from build123d import *

# Parameters (mm, degrees)
SKETCH_1_R          = 2
SKETCH_1_R_2        = 1.5
SKETCH_1_R_3        = 13.75
EXTRUDE_1_DEPTH     = 4
SKETCH1_W           = 111
SKETCH1_H           = 110
SKETCH1_R           = 1.6
SKETCH1_R_2         = 2.1
SKETCH1_R_3         = 25
BOSS_EXTRUDE1_DEPTH = 4
FILLET1_R           = 10
FILLET2_DEPTH       = 4
CUT_EXTRUDE1_DEPTH  = 10


with BuildPart() as part:
    # 草图1 → 凸台-拉伸1 (new body)
    with BuildSketch(Plane(origin=(0, 0, 0), x_dir=(1, 0, 0), z_dir=(0, 1, 0))):
        with BuildLine():
            Line((-43.799718629, 20.922806374), (-13.545390598, 30.755183267))
            ThreePointArc((-13.545390598, 30.755183267), (-12.782331025, 30.938416565), (-12, 31))
            Line((-12, 31), (12, 31))
            ThreePointArc((12, 31), (12.782331025, 30.938416565), (13.545390598, 30.755183267))
            Line((13.545390598, 30.755183267), (43.799718629, 20.922806374))
            ThreePointArc((43.799718629, 20.922806374), (58.729032885, -3.442256511), (37, -22))
            Line((37, -22), (-37, -22))
            ThreePointArc((-37, -22), (-58.729032885, -3.442256511), (-43.799718629, 20.922806374))
        make_face()
        with Locations(Location((-12, 26, 0), (0, 0, 270))):
            Circle(SKETCH_1_R, mode=Mode.SUBTRACT)
        with Locations(Location((12, 26, 0), (0, 0, 270))):
            Circle(SKETCH_1_R, mode=Mode.SUBTRACT)
        with Locations(Location((49.374368671, 12.374368671, 0), (0, 0, 270))):
            Circle(SKETCH_1_R_2, mode=Mode.SUBTRACT)
        with Locations(Location((49.374368671, -12.374368671, 0), (0, 0, 270))):
            Circle(SKETCH_1_R_2, mode=Mode.SUBTRACT)
        with Locations(Location((24.625631329, -12.374368671, 0), (0, 0, 270))):
            Circle(SKETCH_1_R_2, mode=Mode.SUBTRACT)
        with Locations(Location((24.625631329, 12.374368671, 0), (0, 0, 270))):
            Circle(SKETCH_1_R_2, mode=Mode.SUBTRACT)
        with Locations(Location((-49.374368671, -12.374368671, 0), (0, 0, 90))):
            Circle(SKETCH_1_R_2, mode=Mode.SUBTRACT)
        with Locations(Location((-24.625631329, -12.374368671, 0), (0, 0, 90))):
            Circle(SKETCH_1_R_2, mode=Mode.SUBTRACT)
        with Locations(Location((-49.374368671, 12.374368671, 0), (0, 0, 90))):
            Circle(SKETCH_1_R_2, mode=Mode.SUBTRACT)
        with Locations(Location((-24.625631329, 12.374368671, 0), (0, 0, 90))):
            Circle(SKETCH_1_R_2, mode=Mode.SUBTRACT)
        with Locations(Location((-37, 0, 0), (0, 0, 270))):
            Circle(SKETCH_1_R_3, mode=Mode.SUBTRACT)
        with Locations(Location((37, 0, 0), (0, 0, 90))):
            Circle(SKETCH_1_R_3, mode=Mode.SUBTRACT)
    extrude(amount=EXTRUDE_1_DEPTH)

    # Sketch1 → Boss-Extrude1 (add)
    with BuildSketch(Plane(origin=(0, 4, 0), x_dir=(1, 0, 0), z_dir=(0, 1, 0))):
        with Locations((18.5, -77)):
            Rectangle(SKETCH1_W, SKETCH1_H)
        with Locations(Location((12, -34, 0), (0, 0, 270))):
            Circle(SKETCH1_R, mode=Mode.SUBTRACT)
        with Locations(Location((-12, -34, 0), (0, 0, 270))):
            Circle(SKETCH1_R, mode=Mode.SUBTRACT)
        with Locations(Location((-2.941125497, -122.941125497, 0), (0, 0, 270))):
            Circle(SKETCH1_R_2, mode=Mode.SUBTRACT)
        with Locations(Location((64.941125497, -122.941125497, 0), (0, 0, 270))):
            Circle(SKETCH1_R_2, mode=Mode.SUBTRACT)
        with Locations(Location((64.941125497, -55.058874503, 0), (0, 0, 270))):
            Circle(SKETCH1_R_2, mode=Mode.SUBTRACT)
        with Locations(Location((31, -89, 0), (0, 0, 270))):
            Circle(SKETCH1_R_3, mode=Mode.SUBTRACT)
    extrude(amount=-BOSS_EXTRUDE1_DEPTH)

    # Fillet1
    fillet1_edges = [part.edges().sort_by_distance(p)[0] for p in [
        (-37, 2, 22),
        (-37, 2, 132),
        (74, 2, 22),
        (74, 2, 132),
    ]]
    fillet(fillet1_edges, radius=FILLET1_R)

    # Fillet2: read off the stored shape, not the designer's step
    # Fillet2 outline → Fillet2 (add)
    with BuildSketch(Plane(origin=(0, 0, 0), x_dir=(1, 0, 0), z_dir=(0, 1, 0))):
        with BuildLine():
            ThreePointArc((65.297899409, -22.084584874), (57.943895671, -17.183606101), (57.347111687, -8.366304201))
            ThreePointArc((57.347111687, -8.366304201), (49.246250601, -18.276469742), (37, -22))
            Line((37, -22), (64, -22))
            ThreePointArc((64, -22), (64.650326356, -22.021168624), (65.297899409, -22.084584874))
        make_face()
    extrude(amount=FILLET2_DEPTH)

    # Sketch2 → Cut-Extrude1 (cut)
    with BuildSketch(Plane(origin=(0, 4, 0), x_dir=(1, 0, 0), z_dir=(0, 1, 0))):
        with BuildLine():
            Line((-2, 31), (2, 31))
            Line((2, 31), (2, 22.743593539))
            ThreePointArc((2, 22.743593539), (1.560660172, 21.682933368), (0.5, 21.243593539))
            Line((0.5, 21.243593539), (-0.5, 21.243593539))
            ThreePointArc((-0.5, 21.243593539), (-1.560660172, 21.682933368), (-2, 22.743593539))
            Line((-2, 22.743593539), (-2, 31))
        make_face()
        with BuildLine():
            Line((-0.5, -29.243593539), (0.5, -29.243593539))
            ThreePointArc((0.5, -29.243593539), (1.560660172, -29.682933368), (2, -30.743593539))
            Line((2, -30.743593539), (2, -37.5))
            ThreePointArc((2, -37.5), (1.560660172, -38.560660172), (0.5, -39))
            Line((0.5, -39), (-0.5, -39))
            ThreePointArc((-0.5, -39), (-1.560660172, -38.560660172), (-2, -37.5))
            Line((-2, -37.5), (-2, -30.743593539))
            ThreePointArc((-2, -30.743593539), (-1.560660172, -29.682933368), (-0.5, -29.243593539))
        make_face()
    extrude(amount=-CUT_EXTRUDE1_DEPTH, mode=Mode.SUBTRACT)


solid = part.part
Build history of the part. All positions in model axes, mm. A direction names the side the tool comes from. Coordinates: 2 decimals unless noted, no trailing zeros. Order: outer loops, then holes, each group sorted by start corner. A loop starts at its lowest first (then second) coordinate and runs counter-clockwise, first axis right, second up. Notation, with made-up numbers: (9, -28) - (35, -28) arc R21 ccw to (35, -17) - close; hole circle Ø9 at (59.5, -20). An arc over 180 degrees is marked (long way). Write item = value, one per line. Start each with the question number.
1) Wall check: line 1 along X through (y, z) = (2.6, 0); line 2 along Z through (x, y) = (38.5, 3.5); line 3 along Z through (x, y) = (-48.5, 1.4) (3 decimals). Give the ranges that are in metal, low to high. Write a range as from..to.
2) Saw through at C-C on z = -26. Write the cut outline in (x, y), then the cut area to 3 significant figures.
3) Saw through at A-A on z = 89. Write the cut outline in (x, y).
4) Saw through at B-B on x = 37. Write the cut outline in (y, z).
5) Flat gauge pins, fed straight in: pin 1 Ø1.9 at (x, z) = (12, 34) entering from -Y; pin 2 Ø2 at (y, z) = (1, 64) entering from -X; pin 3 Ø1 at (x, y) = (56, 3.5) entering from -Z. Where does each tip first touch, or does it go through?
6) Saw through at D-D on x = -32. Write the cut outline in (y, z), then the cut area to 3 significant figures.
7) Two-plate mould, pull along X, no slides. Class faces 1 (the face through (-38.848, 2.028, 24.606)), 2 (the face through (-2, 2, 34)), 3 (the face through (28.46, 1.97, -25.91)): pulls with the +X half, pulls with the -X half, needs draft (parallel to the pull), parting line crosses it, or undercut.
8) 3-axis set-ups, long thin cutter, end or side, ignore diameter. For faces 4 (the face through (-37, 2, 77)), 5 (the face through (-2, 2, -27)), 6 (the face through (32.099, 2.028, 64.024)): which of +Z, -Z, +X, -X, +Y, -Y reach the whole face in a straight line?
From the geometry:
q1.line_1 = -59..-50.75, -23.25..23.25, 50.75..59
q1.line_2 = -22.65..-13.67, 13.67..65.15, 112.85..132
q1.line_3 = -18.755..-13.593, -11.156..-7.537, 7.537..11.156, 13.593..18.755
q2.outline = (-28.18, 0) - (-14, 0) - (-14, 4) - (-28.18, 4) - close; (-10, 0) - (-2, 0) - (-2, 4) - (-10, 4) - close; (2, 0) - (10, 0) - (10, 4) - (2, 4) - close; (14, 0) - (28.18, 0) - (28.18, 4) - (14, 4) - close
q2.area = 177 mm^2
q3.outline = (-37, 0) - (6, 0) - (6, 4) - (-37, 4) - close; (56, 0) - (74, 0) - (74, 4) - (56, 4) - close
q4.outline = (0, -23.13) - (4, -23.13) - (4, -13.75) - (0, -13.75) - close; (0, 13.75) - (4, 13.75) - (4, 64.73) - (0, 64.73) - close; (0, 113.27) - (4, 113.27) - (4, 132) - (0, 132) - close
q5.pin_1 = through
q5.pin_2 = -37
q5.pin_3 = -11.91
q6.outline = (0, -24.76) - (4, -24.76) - (4, -12.81) - (0, -12.81) - close; (0, 12.81) - (4, 12.81) - (4, 130.66) - (0, 130.66) - close
q6.area = 519 mm^2
q7.face_1 = pulls with the -X half
q7.face_2 = undercut
q7.face_3 = pulls with the +X half
q8.face_4 = +Z, -X, +Y, -Y
q8.face_5 = -Z, +Y, -Y
q8.face_6 = +Y, -Y
